For this review, take the finished solid that the model builds, in its own axes (mm). A direction names the side the tool comes from. Give positions to 0.01 mm unless a question says otherwise; leave off trailing zeros. Loops run counter-clockwise (first coordinate to the right, second up) from the corner with the lowest first, then second, coordinate; pieces in that order, holes last. Notation, with made-up numbers: (22, 26) - (52, 26) arc R12 ccw to (52, 31) - close; hole circle Ø10 at (27.25, 25.5). An arc over 180 degrees is marked (long way). Put each result on its own line as item: value.
from build123d import *
from OCP.BRepFilletAPI import BRepFilletAPI_MakeChamfer

# Parameters (mm, degrees)
SKETCH_2_W          = 250
SKETCH_2_H          = 110
EXTRUDE_1_DEPTH     = 15
SKETCH_3_W          = 235.794340166
SKETCH_3_H          = 96.388664916
CUT_EXTRUDE_1_DEPTH = 5
SKETCH_4_W          = 195.385858248
SKETCH_4_H          = 85.621380658
CUT_EXTRUDE_2_DEPTH = 1
CHAMFER_1_SIZE      = 4
CHAMFER_1_SIZE2     = 3.730060345
SKETCH_6_R          = 5
EXTRUDE_2_DEPTH     = 40


with BuildPart() as part:
    # 草图2 → 凸台-拉伸1 (new body)
    with BuildSketch(Plane.XY):
        Rectangle(SKETCH_2_W, SKETCH_2_H)
    extrude(amount=EXTRUDE_1_DEPTH)

    # 草图3 → 切除-拉伸1 (cut)
    with BuildSketch(Plane.XY.offset(15)):
        Rectangle(SKETCH_3_W, SKETCH_3_H)
    extrude(amount=-CUT_EXTRUDE_1_DEPTH, mode=Mode.SUBTRACT)

    # 草图4 → 切除-拉伸2 (cut)
    with BuildSketch(Plane.XY.offset(10)):
        Rectangle(SKETCH_4_W, SKETCH_4_H)
    extrude(amount=-CUT_EXTRUDE_2_DEPTH, mode=Mode.SUBTRACT)

    # 倒角1: one chamfer whose edges measure the first distance from different faces: ONE call of the kernel's chamfer builder (chamfer() names one face for all edges)
    chamfer_1_edges_1 = [part.edges().sort_by_distance(p)[0] for p in [
        (117.897170083, 0, 15),
        (0, 48.194332458, 15),
        (-117.897170083, 0, 15),
        (0, -48.194332458, 15),
    ]]
    chamfer_1_side_1 = [part.faces().sort_by_distance(p)[0] for p in [
        (0, -52.268699943, 15),
    ]]
    chamfer_1_edges_2 = [part.edges().sort_by_distance(p)[0] for p in [
        (-125, 0, 0),
    ]]
    chamfer_1_side_2 = [part.faces().sort_by_distance(p)[0] for p in [
        (0, 0, 0),
    ]]
    chamfer_1 = BRepFilletAPI_MakeChamfer(part.part.solid().wrapped)
    for e in chamfer_1_edges_1:
        chamfer_1.Add(CHAMFER_1_SIZE, CHAMFER_1_SIZE2, e.wrapped, chamfer_1_side_1[0].wrapped)  # the first distance lies on this face
    for e in chamfer_1_edges_2:
        chamfer_1.Add(CHAMFER_1_SIZE, CHAMFER_1_SIZE2, e.wrapped, chamfer_1_side_2[0].wrapped)  # the first distance lies on this face
    add(Compound.cast(chamfer_1.Shape()), mode=Mode.REPLACE)

    # 草图6 → 凸台-拉伸2 (add)
    with BuildSketch(Plane(origin=(0, 0, 0), x_dir=(-1, 0, 0), z_dir=(0, 0, -1))):
        with Locations((0, 25.093271363)):
            Circle(SKETCH_6_R)
    extrude(amount=EXTRUDE_2_DEPTH)


solid = part.part
1) Insertion check: pin 1 Ø6 at (x, y) = (-50, 34) entering from -Z; pin 2 Ø1 at (x, y) = (45, -37.5) entering from +Z; pin 3 Ø5 at (x, z) = (-68.5, -1.5) entering from -Y. Each pin has a flat end and moves straight along its axis. Give the tip position at first contact, or say it passes through.
Geometry check:
pin 1: stops at z = 0
pin 2: stops at z = 9
pin 3: stops at y = -55
2) Draft analysis for pull direction X (two halves, no side actions). For faces 3 (the face through (0.65, 30.05, -19.72)), 4 (the face through (0, 1, 0)), 5 (the face through (-1, 43, 10)), state which applies: pulls with the +X half, pulls with the -X half, needs draft (parallel to the pull), parting line crosses it, or undercut.
Geometry check:
face 3: parting line crosses it
face 4: needs draft
face 5: undercut
3) Wall thickness on line 1 (Z direction, x = 19, y = 1); line 2 (Z direction, x = -93.5, y = 45.5); line 3 (Y direction, x = 12, z = 13.5): over which ranges is each line inside the solid? List them lowest first.
Geometry check:
line 1: z = 0 to 9
line 2: z = 0 to 10
line 3: y = -55 to -50.59, 50.59 to 55
4) Take a section at B-B on x = -60. State the section outline as (y, z) points, and give its area (3 significant figures).
Geometry check:
outline: (-55, 0) - (55, 0) - (55, 15) - (52.19, 15) - (48.19, 11.27) - (48.19, 10) - (42.81, 10) - (42.81, 9) - (-42.81, 9) - (-42.81, 10) - (-48.19, 10) - (-48.19, 11.27) - (-52.19, 15) - (-55, 15) - close
area: 1,070 mm²
5) Take a section at A-A on y = 17. State the section outline as (x, z) points, and give its area (3 significant figures).
Geometry check:
outline: (-125, 3.73) - (-121, 0) - (125, 0) - (125, 15) - (121.9, 15) - (117.9, 11.27) - (117.9, 10) - (97.69, 10) - (97.69, 9) - (-97.69, 9) - (-97.69, 10) - (-117.9, 10) - (-117.9, 11.27) - (-121.9, 15) - (-125, 15) - close
area: 2,350 mm²
6) Take a section at D-D on x = 0. State the section outline as (y, z) points, and give its area (3 significant figures).
Geometry check:
outline: (-55, 0) - (20.09, 0) - (20.09, -40) - (30.09, -40) - (30.09, 0) - (55, 0) - (55, 15) - (52.19, 15) - (48.19, 11.27) - (48.19, 10) - (42.81, 10) - (42.81, 9) - (-42.81, 9) - (-42.81, 10) - (-48.19, 10) - (-48.19, 11.27) - (-52.19, 15) - (-55, 15) - close
area: 1,470 mm²
7) For faces 1 (the face through (-1, 1, 9)), 2 (the face through (-2, 55, 7)), list the 3-axis set-ups (+Z, -Z, +X, -X, +Y, -Y) from which the entire face can be reached by the end or side of a thin tool; tool diameter is ignored.
Geometry check:
face 1: +Z
face 2: +Z, -Z, +X, -X, +Y
8) Take a section at C-C on z = -4.5. State the section outline as (x, y) points.
Geometry check:
outline: circle Ø10 at (0, 25.09)
